The model under review builds one solid part; all positions refer to its coordinate system, in mm. A direction names the side the tool comes from. Round coordinates to 2 decimals unless told otherwise and drop trailing zeros. Loops run counter-clockwise (first coordinate to the right, second up) from the corner with the lowest first, then second, coordinate; pieces in that order, holes last. Notation, with made-up numbers: (42.25, 26) -> (96.25, 26) arc R13 ccw to (96.25, 39) -> close; hole circle Ø5 at (62, -15). An arc over 180 degrees is marked (long way). Use a Markdown table: item, result. Add a question column.
1) Consider section A-A on y = 116. Give the boundary of the cut face in (x, z) (3 decimals), plus the area to 3 significant figures.
2) Consider section C-C on x = -12.7. State how many separate pieces and enclosed holes the cut face has, plus the area to 3 significant figures.
3) Consider section D-D on y = -4. Give the boundary of the cut face in (x, z), plus the area to 3 significant figures.
4) Wall thickness on probe 1 along Y at (x, z) = (-15, -4.75) (3 decimals); probe 2 along Y at (x, z) = (-22, -4.25) (3 decimals); probe 3 along Y at (x, z) = (-12.7, -0.85) (3 decimals): over which ranges is each line inside the solid? List them lowest first.
5) Mouldability with a two-part tool opening along Y and no side actions: class faces 1 (the flat face through (-13, 65, 0)), 2 (the cylindrical face through (-13.9, 126.6, -18)), 3 (the cylindrical face through (-17.88, 43.935, -1.565)) as released by +Y, released by -Y, zero draft, split by the parting line, or undercut.
6) For faces 4 (the flat face through (-25.4, 62, -1)), 5 (the flat face through (-15, 18, -3.175)), list the 3-axis set-ups (+Z, -Z, +X, -X, +Y, -Y) from which the entire face can be reached by the end or side of a thin tool; tool diameter is ignored.
7) Insertion check: pin 1 (13.5 mm diameter, centred on x = -11, y = -5, fed in from -Z); pin 2 (1.5 mm diameter, centred on x = -11, z = -13.5, fed in from +Y); pin 3 (10.5 mm diameter, centred on x = -14.5, z = -16.5, fed in from -Y); pin 4 (3.5 mm diameter, centred on y = 11, z = -12.5, fed in from +X). Each pin has a flat end and moves straight along its axis. Give the tip position at first contact, or say it passes through.
8) Consider section B-B on y = 24. Give the boundary of the cut face in (x, z) (3 decimals).
from build123d import *

# Parameters (mm, degrees)
BOSS_EXTRUDE1_DEPTH     = 127
CUT_EXTRUDE1_START      = -31.75
CUT_EXTRUDE1_DEPTH      = 28.575
CUT_EXTRUDE2_START      = 31.75
CUT_EXTRUDE2_DEPTH      = 28.575
SKETCH3_W               = 25.4
SKETCH3_H               = 50.8
CUT_EXTRUDE4_DEPTH      = 28.575
SKETCH6_W               = 25.4
SKETCH6_H               = 15.875
SKETCH6_R               = 1.5875
BOSS_EXTRUDE2_DEPTH     = 2.54
CUT_EXTRUDE6_DEPTH      = 148.432177119
CUT_EXTRUDE6_DEPTH_BACK = 148.432177119
SKETCH5_R               = 1.5875
SKETCH7_R               = 2.25
CUT_EXTRUDE7_DEPTH      = 148.514203892
FILLET1_R               = 1.27


with BuildPart() as part:
    # Sketch1 → Boss-Extrude1 (new body)
    with BuildSketch(Plane(origin=(0, 0, 0), x_dir=(1, 0, 0), z_dir=(0, 1, 0))):
        Polygon((0, 0), (-25.4, 0), (-25.4, 6.985), (-3.175, 29.21), (0, 29.21), align=None)
    extrude(amount=BOSS_EXTRUDE1_DEPTH)

    # Sketch2 → Cut-Extrude1 (cut)
    with BuildSketch(Plane(origin=(0, 63.5, 0), x_dir=(-1, 0, 0), z_dir=(0, -1, 0)).offset(CUT_EXTRUDE1_START)):
        Polygon((25.4, 6.985), (3.175, 29.21), (3.175, 3.175), (25.4, 3.175), align=None)
    extrude(amount=-CUT_EXTRUDE1_DEPTH, mode=Mode.SUBTRACT)

    # Sketch2<2> → Cut-Extrude2 (cut)
    with BuildSketch(Plane(origin=(0, 63.5, 0), x_dir=(-1, 0, 0), z_dir=(0, -1, 0)).offset(CUT_EXTRUDE2_START)):
        Polygon((25.4, 6.985), (3.175, 29.21), (3.175, 3.175), (25.4, 3.175), align=None)
    extrude(amount=CUT_EXTRUDE2_DEPTH, mode=Mode.SUBTRACT)

    # Sketch3 → Cut-Extrude4 (cut, symmetric)
    with BuildSketch(Plane(origin=(0, 63.5, 0), x_dir=(-1, 0, 0), z_dir=(0, -1, 0))):
        with Locations((12.7, 28.575)):
            Rectangle(SKETCH3_W, SKETCH3_H)
    extrude(amount=CUT_EXTRUDE4_DEPTH, both=True, mode=Mode.SUBTRACT)

    # Sketch6 → Boss-Extrude2 (add)
    # profile 1 of 2: a face of its own
    with BuildSketch(Plane.XY):
        with Locations((-12.7, 134.9375)):
            Rectangle(SKETCH6_W, SKETCH6_H)
        with Locations((-12.7, 134.9375)):
            Circle(SKETCH6_R, mode=Mode.SUBTRACT)
    # profile 2 of 2: a face of its own
    with BuildSketch(Plane.XY):
        with Locations((-12.7, -7.9375)):
            Rectangle(SKETCH6_W, SKETCH6_H)
        with Locations(Location((-12.7, -7.9375, 0), (0, 0, 180))):
            Circle(SKETCH6_R, mode=Mode.SUBTRACT)
    extrude(amount=-BOSS_EXTRUDE2_DEPTH)

    # Sketch5 → Cut-Extrude6 (cut, two sides: drawn at the far end of the back side and taken through both)
    with BuildSketch(Plane(origin=(0, 0, -3.175), x_dir=(-1, 0, 0), z_dir=(0, 0, -1)).offset(-CUT_EXTRUDE6_DEPTH_BACK)):
        with Locations((6.35, 84.1375)):
            Circle(SKETCH5_R)
        with Locations((19.05, 42.8625)):
            Circle(SKETCH5_R)
    extrude(amount=CUT_EXTRUDE6_DEPTH + CUT_EXTRUDE6_DEPTH_BACK, mode=Mode.SUBTRACT)

    # Sketch7 → Cut-Extrude7 (cut, through all)
    with BuildSketch(Plane.ZY.offset(3.175)):
        with Locations((-12.49625182, 11)):
            Circle(SKETCH7_R)
        with Locations((-12.49625182, 116)):
            Circle(SKETCH7_R)
    extrude(amount=-CUT_EXTRUDE7_DEPTH, mode=Mode.SUBTRACT)

    # Fillet1
    fillet1_edges = [part.edges().sort_by_distance(p)[0] for p in [
        (-14.2875, 127, -18.0975),
        (-25.4, 127, -4.7625),
        (-3.175, 109.5375, -3.175),
        (-3.175, 95.25, -16.1925),
        (-14.2875, 95.25, -3.175),
        (-14.2875, 123.825, -3.175),
        (-3.175, 123.825, -16.1925),
        (-3.175, 31.75, -16.1925),
        (-3.175, 17.4625, -3.175),
        (-14.2875, 31.75, -3.175),
        (-3.175, 3.175, -16.1925),
        (-14.2875, 3.175, -3.175),
        (0, 17.4625, -29.21),
        (-1.5875, 34.925, -29.21),
        (-1.5875, 92.075, -29.21),
        (-25.4, 92.075, -5.08),
        (0, 92.075, -16.1925),
        (-25.4, 34.925, -5.08),
        (-14.2875, 34.925, -18.0975),
        (0, 34.925, -16.1925),
        (-14.2875, 92.075, -18.0975),
        (0, 127, -15.875),
        (-14.2875, 0, -18.0975),
        (0, 142.875, -1.27),
        (-25.4, 142.875, -1.27),
        (-1.5875, 0, -29.21),
        (0, 0, -15.875),
        (0, -15.875, -1.27),
        (-25.4, -15.875, -1.27),
        (-1.5875, 127, -29.21),
        (0, 109.5375, -29.21),
    ]]
    fillet(fillet1_edges, radius=FILLET1_R)


solid = part.part
Result set:
| question | item | result |
|---|---|---|
| 1 | outline | (-25.4, -3.175) -> (-4.445, -3.175) arc R1.27 cw to (-3.175, -4.445) -> (-3.175, -10.246) -> (0, -10.246) -> (0, 0) -> (-25.4, 0) -> close; (-3.175, -29.21) -> (-1.27, -29.21) arc R1.27 ccw to (0, -27.94) -> (0, -14.746) -> (-3.175, -14.746) -> close |
| 1 | area | 149 mm2 |
| 2 | separate pieces | 3 |
| 2 | enclosed holes | 0 |
| 2 | area | 677 mm2 |
| 3 | outline | (-25.4, -2.54) -> (0, -2.54) -> (0, 0) -> (-25.4, 0) -> close |
| 3 | area | 64.5 mm2 |
| 4 | probe 1 | 0 to 3.175, 31.75 to 34.925, 92.075 to 95.25, 123.825 to 127 |
| 4 | probe 2 | 0 to 3.19, 31.735 to 34.925, 92.075 to 95.265, 123.81 to 127 |
| 4 | probe 3 | -15.875 to -9.525, -6.35 to 133.35, 136.525 to 142.875 |
| 5 | face 1 | zero draft |
| 5 | face 2 | released by +Y |
| 5 | face 3 | undercut |
| 6 | face 4 | +Z, -Z, -X, +Y, -Y |
| 6 | face 5 | -Z, -X |
| 7 | pin 1 | z = -24.95 |
| 7 | pin 2 | y = 127 |
| 7 | pin 3 | y = 0 |
| 7 | pin 4 | through |
| 8 | outline | (-25.4, -3.175) -> (-4.445, -3.175) arc R1.27 cw to (-3.175, -4.445) -> (-3.175, -29.21) -> (-1.27, -29.21) arc R1.27 ccw to (0, -27.94) -> (0, 0) -> (-25.4, 0) -> close |
